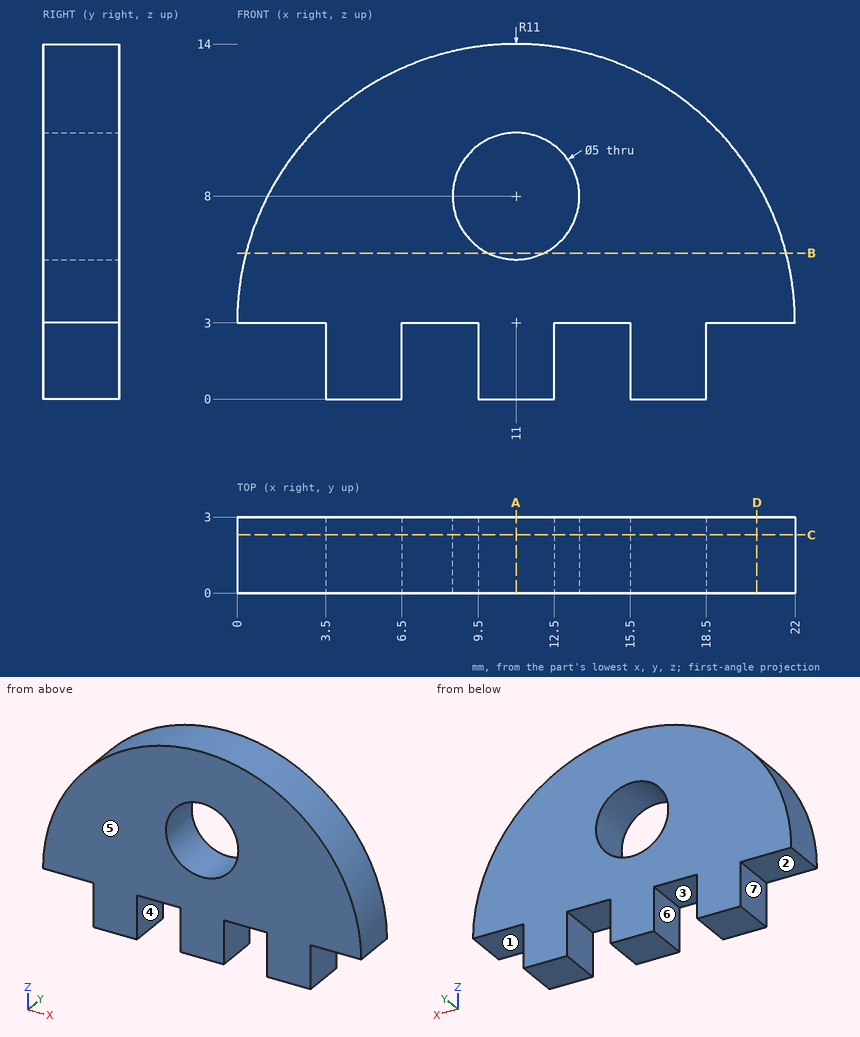
Geometry: see drawing. Coordinates: mm, zero at the bounding-box minimum. A direction names the side the tool comes from. Coordinates: 2 decimals unless noted, no trailing zeros. Loops run counter-clockwise (first coordinate to the right, second up) from the corner with the lowest first, then second, coordinate; pieces in that order, holes last. Notation, with made-up numbers: (41.25, 55) - (54.25, 55) arc R23 cw to (54.25, 87) - close; hole circle Ø2 at (-12.75, -14). An arc over 180 degrees is marked (long way). Put each result on its own line as item: value. Start each with the question number.
Q1. Pull-direction query (X, two-part tool) for the marked faces 4, 5, 6 and 7; classes: released by +X, released by -X, zero draft, split by the parting line, or undercut.
Q2. Cut plane D-D, the plane x = 20.5. Return loops of the section in (y, z), and give its area (3 significant figures).
Q3. Line query: line 1 (Z direction, x = 11, y = 1.6); line 2 (Z direction, x = 9, y = 0.2); line 3 (X direction, y = 2, z = 3.25). Output: solid intervals per line, ascending.
Q4. Cut plane A-A, the plane x = 11. Return loops of the section in (y, z).
Q5. Cut plane B-B, the plane z = 5.75. Return loops of the section in (x, y).
Q6. Pin query (flat end, axial travel): pin 1 Ø1.5 at (x, y) = (21, 1) entering from -Z; pin 2 Ø1 at (y, z) = (0.5, 5) entering from +X; pin 3 Ø3 at (x, z) = (11, 8) entering from -Y; pin 4 Ø1.5 at (y, z) = (1.5, 1) entering from +X. Return the tip coordinate at first contact, or that it passes through.
Q7. Set-up query: the marked faces 1, 2 and 3. Return all of +Z, -Z, +X, -X, +Y, -Y with unobstructed straight access to the full face (end or side cutting, diameter ignored); none if empty.
Q8. Cut plane C-C, the plane y = 2.3. Return loops of the section in (x, z).
Filled sheet:
1. face 4: undercut
1. face 5: zero draft
1. face 6: undercut
1. face 7: released by -X
2. outline: (0, 3) - (3, 3) - (3, 8.55) - (0, 8.55) - close
2. area: 16.6 mm²
3. line 1: 0 to 5.5, 10.5 to 14
3. line 2: 3 to 6.5, 9.5 to 13.82
3. line 3: 0 to 22
4. outline: (0, 0) - (3, 0) - (3, 5.5) - (0, 5.5) - close; (0, 10.5) - (3, 10.5) - (3, 14) - (0, 14) - close
5. outline: (0.35, 0) - (9.91, 0) - (9.91, 3) - (0.35, 3) - close; (12.09, 0) - (21.65, 0) - (21.65, 3) - (12.09, 3) - close
6. pin 1: z = 3
6. pin 2: x = 21.9
6. pin 3: through
6. pin 4: x = 18.5
7. face 1: -Z, +X, +Y, -Y
7. face 2: -Z, -X, +Y, -Y
7. face 3: -Z, +Y, -Y
8. outline: (0, 3) - (3.5, 3) - (3.5, 0) - (6.5, 0) - (6.5, 3) - (9.5, 3) - (9.5, 0) - (12.5, 0) - (12.5, 3) - (15.5, 3) - (15.5, 0) - (18.5, 0) - (18.5, 3) - (22, 3) arc R11 ccw to start; hole circle Ø5 at (11, 8)
